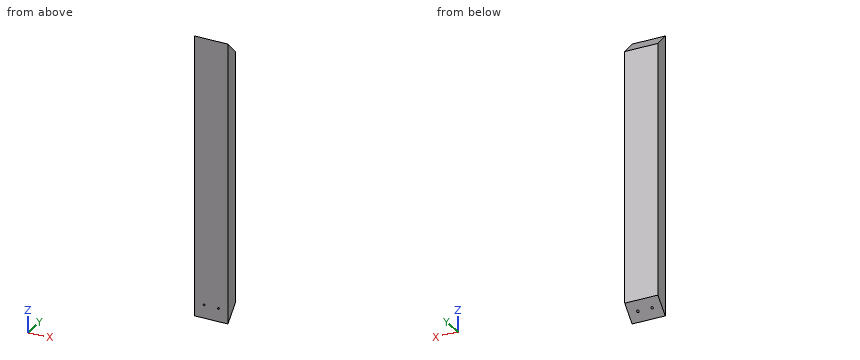
Autodesk Inventor part; units mm, degrees
ref_plane "YZ Plane" through (0, 0, 0) normal (1, 0, 0) x (0, 1, 0)
ref_plane "XZ Plane" through (0, 0, 0) normal (0, 1, 0) x (-1, 0, 0)
ref_plane "XY Plane" through (0, 0, 0) normal (0, 0, 1) x (1, 0, 0)
sketch "Sketch1" plane through (0, 0, 0) normal (1, 0, 0) x (0, 1, 0)
  line L0 (38.1, -38.1) -> (38.1, -717.55)
  line L1 (0, -755.65) -> (0, 0)
  line L2 (0, 0) -> (38.1, -38.1)
  line L3 (0, 0) -> (78.5772, 0) construction
  line L4 (0, -755.65) -> (38.1, -717.55)
  dimension "d2" = 45
  dimension "d20" = 755.65
extrude "Extrusion1" add sketch "Sketch1" along normal blind 88.9
sketch "Sketch2" plane through (88.9, 38.1, -717.55) normal (0, 0.7071, -0.7071) x (-1, 0, 0)
  line L0 (0, -53.8815) -> (0, 0)
  line L1 (88.9, -53.8815) -> (0, -53.8815)
  circle A0 centre (25.4, -26.9408) radius 4.5233
  circle A1 centre (63.5, -26.9408) radius 4.5233
  point P0 (88.9, 480.4437)
  dimension "d5" = 25.4
  dimension "d8" = 38.1
hole "Hole1" at (63.5, 19.05, -736.6) at (25.4, 19.05, -736.6) direction (0, -0.7071, 0.7071) diameter 6.35 depth 25.4 tip angle 118
properties part number "2p2ps45" material "Wood (Cherry)"
The model under review builds one solid part; all positions refer to its coordinate system, in mm. Coordinates: 2 decimals unless noted, no trailing zeros. Write each loop counter-clockwise with the first axis right and the second up, starting at its lowest first coordinate (ties: lowest second). Pieces come first, ordered by that corner, then holes. Notation, with made-up numbers: (36, -26.75) - (52, -26.75) arc R13 cw to (52, -3.75) - close; hole circle Ø10 at (57, 2.5). An arc over 180 degrees is marked (long way). Answer in a Markdown table with one row per item. Add a question column.
Q1. Clearance check with flat-ended pins moving along their axes: pin 1 (1.5 mm diameter, centred on y = 29, z = -408.5, fed in from -X); pin 2 (6 mm diameter, centred on x = 51, y = 18.5, fed in from -Z); pin 3 (4 mm diameter, centred on x = 53.5, y = 7.5, fed in from +Z); pin 4 (2 mm diameter, centred on x = 79.5, y = 17, fed in from -Z). State where each tip first meets the part, or that it passes through.
Q2. Consider section A-A on y = 31. Give the boundary of the cut face in (x, z).
Q3. To check wall thickness, follow line 1 along Z through (x, y) = (27.5, 2.5); line 2 along Z through (x, y) = (28, 12); line 3 along Z through (x, y) = (12, 3). State the ranges of each line that lie inside material, in increasing order. Write a range as from..to.
Q4. Consider section B-B on x = 37.5. Give the boundary of the cut face in (y, z).
Answers below:
| question | item | result |
|---|---|---|
| 1 | pin 1 | x = 0 |
| 1 | pin 2 | z = -740.15 |
| 1 | pin 3 | z = -5.5 |
| 1 | pin 4 | z = -739.65 |
| 2 | outline | (0, -724.65) - (88.9, -724.65) - (88.9, -31) - (0, -31) - close |
| 3 | line 1 | -753.15..-723.42, -717.06..-2.5 |
| 3 | line 2 | -743.65..-732.13, -726.97..-12 |
| 3 | line 3 | -752.65..-3 |
| 4 | outline | (0, -755.65) - (38.1, -717.55) - (38.1, -38.1) - (0, 0) - close |
